```python
from build123d import *

# Parameters (mm, degrees)
SKETCH1_W                 = 279.4
SKETCH1_H                 = 76.2
BOSS_EXTRUDE1_DEPTH       = 3
SKETCH3_W                 = 3
SKETCH3_H                 = 15
SKETCH3_H_2               = 7.8
CUT_EXTRUDE1_DEPTH        = 145.833352512
LPATTERN1_COUNT           = 4
LPATTERN1_PITCH           = 22.8
MIRROR1_COPY_1_SKETCH_W   = 3
MIRROR1_COPY_1_SKETCH_H   = 15
MIRROR1_COPY_1_SKETCH_H_2 = 7.8
MIRROR1_COPY_1_DEPTH      = 145.833352512
MIRROR1_COPY_2_SKETCH_W   = 3
MIRROR1_COPY_2_SKETCH_H   = 15
MIRROR1_COPY_2_SKETCH_H_2 = 7.8
MIRROR1_COPY_2_DEPTH      = 145.833352512
MIRROR1_COPY_3_SKETCH_W   = 3
MIRROR1_COPY_3_SKETCH_H   = 15
MIRROR1_COPY_3_SKETCH_H_2 = 7.8
MIRROR1_COPY_3_DEPTH      = 145.833352512


with BuildPart() as part:
    # Sketch1 → Boss-Extrude1 (new body)
    with BuildSketch(Plane(origin=(0, 0, 0), x_dir=(0, 0, -1), z_dir=(1, 0, 0))):
        Rectangle(SKETCH1_W, SKETCH1_H)
    extrude(amount=-BOSS_EXTRUDE1_DEPTH)

    # Sketch3 → Cut-Extrude1 (cut, through all)
    with BuildSketch(Plane.ZY.offset(3)):
        with Locations((-102.15, 22.8)):
            Rectangle(SKETCH3_W, SKETCH3_H)
        with Locations((-138.2, 34.2)):
            Rectangle(SKETCH3_W, SKETCH3_H_2)
    cut_extrude1 = extrude(amount=-CUT_EXTRUDE1_DEPTH, mode=Mode.SUBTRACT)

    # LPattern1: Cut-Extrude1 ×4
    with Locations(*[(0, -i * LPATTERN1_PITCH, 0) for i in range(1, LPATTERN1_COUNT)]):
        add(cut_extrude1, mode=Mode.SUBTRACT)

    # Mirror1: Cut-Extrude1 across plane
    add(cut_extrude1.mirror(Plane.XY), mode=Mode.SUBTRACT)

    # Mirror1 copy 1 sketch → Mirror1 copy 1 (cut, through all)
    with BuildSketch(Plane(origin=(-3, -22.8, 0), x_dir=(0, 0, -1), z_dir=(-1, 0, 0))):
        with Locations((-102.15, -22.8)):
            Rectangle(MIRROR1_COPY_1_SKETCH_W, MIRROR1_COPY_1_SKETCH_H)
        with Locations((-138.2, -34.2)):
            Rectangle(MIRROR1_COPY_1_SKETCH_W, MIRROR1_COPY_1_SKETCH_H_2)
    extrude(amount=-MIRROR1_COPY_1_DEPTH, mode=Mode.SUBTRACT)

    # Mirror1 copy 2 sketch → Mirror1 copy 2 (cut, through all)
    with BuildSketch(Plane(origin=(-3, -45.6, 0), x_dir=(0, 0, -1), z_dir=(-1, 0, 0))):
        with Locations((-102.15, -22.8)):
            Rectangle(MIRROR1_COPY_2_SKETCH_W, MIRROR1_COPY_2_SKETCH_H)
        with Locations((-138.2, -34.2)):
            Rectangle(MIRROR1_COPY_2_SKETCH_W, MIRROR1_COPY_2_SKETCH_H_2)
    extrude(amount=-MIRROR1_COPY_2_DEPTH, mode=Mode.SUBTRACT)

    # Mirror1 copy 3 sketch → Mirror1 copy 3 (cut, through all)
    with BuildSketch(Plane(origin=(-3, -68.4, 0), x_dir=(0, 0, -1), z_dir=(-1, 0, 0))):
        with Locations((-102.15, -22.8)):
            Rectangle(MIRROR1_COPY_3_SKETCH_W, MIRROR1_COPY_3_SKETCH_H)
        with Locations((-138.2, -34.2)):
            Rectangle(MIRROR1_COPY_3_SKETCH_W, MIRROR1_COPY_3_SKETCH_H_2)
    extrude(amount=-MIRROR1_COPY_3_DEPTH, mode=Mode.SUBTRACT)


solid = part.part
```
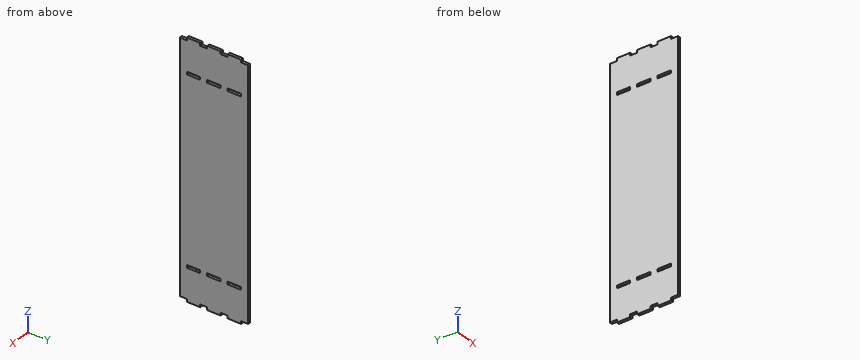
Check sheet for the modelled part. Datum: model origin and axes. Units: mm. Round coordinates to 2 decimals unless told otherwise and drop trailing zeros. Order: outer loops, then holes, each group sorted by start corner. A loop starts at its lowest first (then second) coordinate and runs counter-clockwise, first axis right, second up. Notation, with made-up numbers: (32, 3.25) -> (67, 3.25) arc R17 ccw to (67, 23.25) -> close; hole circle Ø10 at (7, -3.5). An arc over 180 degrees is marked (long way). One line per item, written item: value. Start each with the question number.
Q1. Gauge pin test, flat ends, axial feed: pin 1 Ø12 at (y, z) = (-9.5, -16) entering from +X; pin 2 Ø1.5 at (x, z) = (-1, -138) entering from +Y; pin 3 Ø0.9 at (x, z) = (-2, 138) entering from -Y. Record the tip position at first contact, or that the pin passes through.
Q2. Cross-section at A-A (y = -24). Record the boundary of the cut face in (x, z).
Q3. Cross-section at C-C (y = 33). Record the boundary of the cut face in (x, z), and give its area (3 significant figures).
Q4. Cross-section at B-B (x = -1.4). Give the number of separate pieces and of enclosed holes in the cut face, and give its area (3 significant figures).
Q5. Thickness scan on line 1 (Z direction, x = -0.45, y = -15.5); line 2 (Z direction, x = -1.1, y = 13). Record the ranges inside material, lowest first.
Completed:
1. pin 1: stops at x = 0
1. pin 2: stops at y = 30.3
1. pin 3: stops at y = -30.3
2. outline: (-3, -139.7) -> (0, -139.7) -> (0, -103.65) -> (-3, -103.65) -> close; (-3, -100.65) -> (0, -100.65) -> (0, 100.65) -> (-3, 100.65) -> close; (-3, 103.65) -> (0, 103.65) -> (0, 139.7) -> (-3, 139.7) -> close
3. outline: (-3, -136.7) -> (0, -136.7) -> (0, 136.7) -> (-3, 136.7) -> close
3. area: 820 mm²
4. separate pieces: 1
4. enclosed holes: 6
4. area: 20,800 mm²
5. line 1: z = -139.7 to -103.65, -100.65 to 100.65, 103.65 to 139.7
5. line 2: z = -136.7 to 136.7
